Build history of the part. All positions in model axes, mm. Face numbers are marked on the shaded views. A direction names the side the tool comes from. Give positions to 0.01 mm unless a question says otherwise; leave off trailing zeros. Loops run counter-clockwise (first coordinate to the right, second up) from the corner with the lowest first, then second, coordinate; pieces in that order, holes last. Notation, with made-up numbers: (-23, -6.75) - (16, -6.75) arc R25 ccw to (16, 24.25) - close; hole circle Ø8 at (-15.75, -17.75). An arc over 180 degrees is marked (long way). Return JSON: item names as keys, results as strings. Group by question number.
1) Slice it at B-B (y = 0). Count the separate pieces of the cut face and the enclosed holes in it, and give its area (3 significant figures).
2) 3-axis set-ups, long thin cutter, end or side, ignore diameter. For the marked faces 1, 2, 3, 4 and 5: which of +Z, -Z, +X, -X, +Y, -Y reach the whole face in a straight line?
3) Slice it at A-A (z = 2.75). List the corners of the cut face in (x, y), and give its area (3 significant figures).
4) Slice it at D-D (y = -4). List the corners of the cut face in (x, z).
5) Drop flat-ended pins along their axis: pin 1 (0.8 mm diameter, centred on y = -12, z = 1, fed in from +X); pin 2 (1.5 mm diameter, centred on y = -0.5, z = 1, fed in from +X); pin 3 (2 mm diameter, centred on y = -9, z = -0.5, fed in from -X); pin 4 (1.5 mm diameter, centred on y = -0.5, z = -0.5, fed in from +X). Give the stop position or say it passes through.
6) Drill centre lines: probe 1 along Y at (x, z) = (0, 3.3); probe 2 along Z at (x, y) = (-4.75, -1.5); probe 3 along Y at (x, z) = (8, 0.5). Where is each one in solid material? Low to high. Write a range as from..to.
7) Mould opens along X. For the marked faces 6, 7, 8 and 9 say: released by +X, released by -X, zero draft, split by the parting line, or undercut.
```python
from build123d import *
from OCP.BRepFilletAPI import BRepFilletAPI_MakeChamfer

# Parameters (mm, degrees)
BOSS_EXTRUDE1_DEPTH      = 4.5
BOSS_EXTRUDE1_DEPTH_BACK = 4.5
CUT_EXTRUDE1_START       = -6.1
CUT_EXTRUDE1_DEPTH       = 3.2
CUT_EXTRUDE2_DEPTH       = 19.277658975
CUT_EXTRUDE2_DEPTH_BACK  = 19.277658975
SKETCH3_R                = 1.6
SKETCH4_W                = 20
SKETCH4_H                = 4.97497426
CUT_EXTRUDE3_DEPTH       = 2
SKETCH5_W                = 20
SKETCH5_H                = 5.22601356
CUT_EXTRUDE4_DEPTH       = 2
FILLET1_R                = 0.25
CHAMFER1_SIZE            = 0.5
CHAMFER1_SIZE2           = 0.368761208
CHAMFER2_SIZE            = 0.5


with BuildPart() as part:
    # Sketch1 → Boss-Extrude1 (new, two sides: drawn at the far end of the back side and taken through both)
    with BuildSketch(Plane.XY.offset(-BOSS_EXTRUDE1_DEPTH_BACK)):
        with BuildLine():
            Line((-10, -8.141956011), (-4.311694326, 2.339879755))
            ThreePointArc((-4.311694326, 2.339879755), (0, 4.905684991), (4.311694326, 2.339879755))
            Line((4.311694326, 2.339879755), (10, -8.141956011))
            Line((10, -8.141956011), (0, -8.141956011))
            Line((0, -8.141956011), (0, -10.141956011))
            Line((0, -10.141956011), (4, -10.141956011))
            ThreePointArc((4, -10.141956011), (5.5, -9.911652018), (7, -10.141956011))
            Line((7, -10.141956011), (7, -10.891956011))
            Line((7, -10.891956011), (4, -10.891956011))
            Line((4, -10.891956011), (4, -11.391956011))
            Line((4, -11.391956011), (7, -11.391956011))
            Line((7, -11.391956011), (7, -12.141956011))
            ThreePointArc((7, -12.141956011), (5.5, -12.372260004), (4, -12.141956011))
            Line((4, -12.141956011), (-5, -12.141956011))
            Line((-5, -12.141956011), (-5, -8.141956011))
            Line((-5, -8.141956011), (-10, -8.141956011))
        make_face()
    extrude(amount=BOSS_EXTRUDE1_DEPTH + BOSS_EXTRUDE1_DEPTH_BACK)

    # Sketch2 → Cut-Extrude1 (cut)
    with BuildSketch(Plane.XY.offset(4.5).offset(CUT_EXTRUDE1_START)):
        with BuildLine():
            Line((8.566257505, -5.5), (4.311694326, 2.339879755))
            ThreePointArc((4.311694326, 2.339879755), (0, 4.905684991), (-4.311694326, 2.339879755))
            Line((-4.311694326, 2.339879755), (-8.566257505, -5.5))
            Line((-8.566257505, -5.5), (8.566257505, -5.5))
        make_face()
    extrude(amount=CUT_EXTRUDE1_DEPTH, mode=Mode.SUBTRACT)

    # Sketch3 → Cut-Extrude2 (cut, two sides: drawn at the far end of the back side and taken through both)
    with BuildSketch(Plane.XY.offset(4.5).offset(-CUT_EXTRUDE2_DEPTH_BACK)):
        Circle(SKETCH3_R)
    extrude(amount=CUT_EXTRUDE2_DEPTH + CUT_EXTRUDE2_DEPTH_BACK, mode=Mode.SUBTRACT)

    # Sketch4 → Cut-Extrude3 (cut)
    with BuildSketch(Plane.XY.offset(4.5)):
        with Locations((0, -10.629443141)):
            Rectangle(SKETCH4_W, SKETCH4_H)
    extrude(amount=-CUT_EXTRUDE3_DEPTH, mode=Mode.SUBTRACT)

    # Sketch5 → Cut-Extrude4 (cut)
    with BuildSketch(Plane(origin=(0, 0, -4.5), x_dir=(-1, 0, 0), z_dir=(0, 0, -1))):
        with Locations((0, -10.754962791)):
            Rectangle(SKETCH5_W, SKETCH5_H)
    extrude(amount=-CUT_EXTRUDE4_DEPTH, mode=Mode.SUBTRACT)

    # Fillet1
    fillet1_edges = [part.edges().sort_by_distance(p)[0] for p in [
        (4, -11.391956011, 0),
        (4, -10.891956011, 0),
    ]]
    fillet(fillet1_edges, radius=FILLET1_R - 0.0001)  # a hair under: the kernel refuses the full size

    # Chamfer1: one chamfer whose edges measure the first distance from different faces: ONE call of the kernel's chamfer builder (chamfer() names one face for all edges)
    chamfer1_edges_1 = [part.edges().sort_by_distance(p)[0] for p in [
        (-10, -8.141956011, 0),
    ]]
    chamfer1_side_1 = [part.faces().sort_by_distance(p)[0] for p in [
        (0.403225806, -8.141956011, 0),
    ]]
    chamfer1_edges_2 = [part.edges().sort_by_distance(p)[0] for p in [
        (10, -8.141956011, 0),
    ]]
    chamfer1_side_2 = [part.faces().sort_by_distance(p)[0] for p in [
        (4.382957635, 2.20856292, 3.05),
    ]]
    chamfer1_edges_3 = [part.edges().sort_by_distance(p)[0] for p in [
        (7.155847163, -2.901038128, -4.5),
        (0, 4.905684991, -4.5),
        (7.155847163, -2.901038128, 4.5),
        (0, 4.905684991, 4.5),
        (-7.155847163, -2.901038128, 4.5),
        (-7.155847163, -2.901038128, -4.5),
        (0, 4.905684991, -1.6),
        (6.438975915, -1.580060123, -1.6),
        (-6.438975915, -1.580060123, -1.6),
        (0, 4.905684991, 1.6),
        (-6.438975915, -1.580060123, 1.6),
        (6.438975915, -1.580060123, 1.6),
        (-1.6, 0, 1.6),
        (-1.6, 0, 4.5),
        (-1.6, 0, -1.6),
        (-1.6, 0, -4.5),
    ]]
    chamfer1 = BRepFilletAPI_MakeChamfer(part.part.solid().wrapped)
    for e in chamfer1_edges_1:
        chamfer1.Add(CHAMFER1_SIZE, CHAMFER1_SIZE2, e.wrapped, chamfer1_side_1[0].wrapped)  # the first distance lies on this face
    for e in chamfer1_edges_2:
        chamfer1.Add(CHAMFER1_SIZE, CHAMFER1_SIZE2, e.wrapped, chamfer1_side_2[0].wrapped)  # the first distance lies on this face
    for e in chamfer1_edges_3:
        chamfer1.Add(CHAMFER1_SIZE, e.wrapped)
    add(Compound.cast(chamfer1.Shape()), mode=Mode.REPLACE)

    # Chamfer2
    chamfer2_edges = [part.edges().sort_by_distance(p)[0] for p in [
        (-5, -10.141956011, 2.5),
        (0, -9.141956011, 2.5),
        (2, -10.141956011, 2.5),
        (5.5, -9.911652018, 2.5),
        (5.5, -12.372260004, 2.5),
        (-0.5, -12.141956011, 2.5),
        (-5, -12.141956011, 0),
        (0, -9.141956011, -2.5),
        (2, -10.141956011, -2.5),
        (5.5, -9.911652018, -2.5),
        (5.5, -12.372260004, -2.5),
        (-0.5, -12.141956011, -2.5),
        (-5, -10.141956011, -2.5),
    ]]
    chamfer(chamfer2_edges, length=CHAMFER2_SIZE)


solid = part.part
```
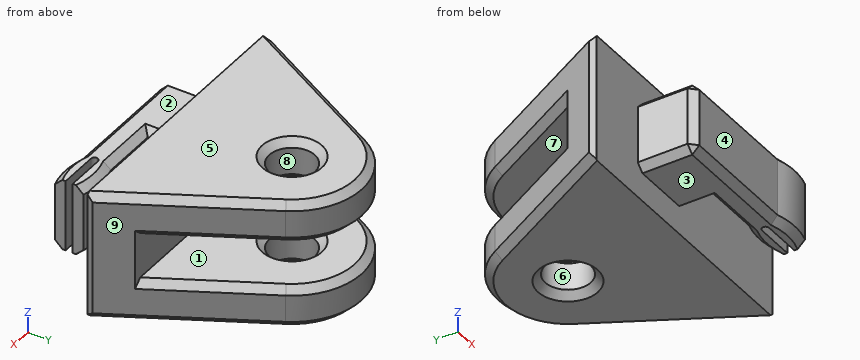
Results:
{
 "1": {"separate pieces": "4", "enclosed holes": "0", "area": "44.0 mm2"},
 "2": {"face 1": "+X, -X, +Y", "face 2": "+Z, +X, -X, -Y", "face 3": "-Z, +X, -X, -Y", "face 4": "+Z, -Z, -X, -Y", "face 5": "+Z, +X, -X, +Y, -Y"},
 "3": {"outline": "(-9.82, -7.82) - (-9.5, -8.14) - (9.63, -8.14) - (9.76, -7.7) - (4.31, 2.34) arc R4.91 ccw to (-4.31, 2.34) - close; hole circle Ø3.2 at (0, 0)", "area": "158 mm2"},
 "4": {"outline": "(-7.75, -4) - (-7.18, -4.5) - (7.18, -4.5) - (7.75, -4) - (7.75, -2.1) - (7.18, -1.6) - (-7.18, -1.6) - (-7.75, -2.1) - close; (-7.75, 2.1) - (-7.18, 1.6) - (7.18, 1.6) - (7.75, 2.1) - (7.75, 4) - (7.18, 4.5) - (-7.18, 4.5) - (-7.75, 4) - close"},
 "5": {"pin 1": "x = 7", "pin 2": "x = 5.55", "pin 3": "x = -9.64", "pin 4": "through"},
 "6": {"probe 1": "-8.14..-1.6, 1.6..4.91", "probe 2": "-4.5..-1.6, 1.6..4.5", "probe 3": "-8.14..-5.5"},
 "7": {"face 6": "undercut", "face 7": "zero draft", "face 8": "undercut", "face 9": "released by +X"}
}
